Part model, mm, in its own coordinate system. Give positions to 0.01 mm unless a question says otherwise; leave off trailing zeros. Write each loop counter-clockwise with the first axis right and the second up, starting at its lowest first coordinate (ties: lowest second). Pieces come first, ordered by that corner, then holes. Notation, with made-up numbers: M 71.5,-19.75 L 78.5,-19.75 A29 cw 78.5,0.25 Z; hole C -18.5,81 d10. An arc over 180 degrees is marked long. Use CSV: the item, a comma, the result in double quotes. Start each with the question number.
1. Drop a flat-ended pin along its axis: pin 1 Ø3.5 at (x, z) = (-87.1, -54.87) entering from +Y. Give the stop position or say it passes through.
2. Band-saw the part on B-B, the plane x = -20. List the corners of the cut face in (y, z), then the cut area to 3 significant figures.
3. Drill centre lines: line 1 along Z through (x, y) = (71, 1.7); line 2 along X through (y, z) = (5, 5). Where is each one in solid material? Low to high. Write a range as from..to.
4. Band-saw the part on A-A, the plane z = -29.5. List the corners of the cut face in (x, y), then the cut area to 3 significant figures.
5. Band-saw the part on C-C, the plane y = 1.9. List the corners of the cut face in (x, z).
from build123d import *

# Parameters (mm, degrees)
SKETCH_1_W          = 187
SKETCH_1_H          = 114
EXTRUDE_1_DEPTH     = 6
FILLET_1_R          = 3
SKETCH_3_W          = 164.9
SKETCH_3_H          = 101.6
CUT_EXTRUDE_1_DEPTH = 6
SKETCH_6_R          = 1.5
CUT_EXTRUDE_3_DEPTH = 6
SKETCH_7_R          = 2.75
CUT_EXTRUDE_4_DEPTH = 2


with BuildPart() as part:
    # 草图1 → 凸台-拉伸1 (new body)
    with BuildSketch(Plane(origin=(0, 0, 0), x_dir=(1, 0, 0), z_dir=(0, 1, 0))):
        with Locations((0.200214133, 4.065310493)):
            Rectangle(SKETCH_1_W, SKETCH_1_H)
    extrude(amount=EXTRUDE_1_DEPTH)

    # 圆角1
    fillet_1_edges = [part.edges().sort_by_distance(p)[0] for p in [
        (-93.299785867, 3, -61.065310493),
        (93.700214133, 3, -61.065310493),
        (93.700214133, 3, 52.934689507),
        (-93.299785867, 3, 52.934689507),
    ]]
    fillet(fillet_1_edges, radius=FILLET_1_R)

    # 草图3 → 切除-拉伸1 (cut)
    with BuildSketch(Plane(origin=(0, 6, 0), x_dir=(1, 0, 0), z_dir=(0, 1, 0))):
        with Locations((0.200562113, 4.065310493)):
            Rectangle(SKETCH_3_W, SKETCH_3_H)
    extrude(amount=-CUT_EXTRUDE_1_DEPTH, mode=Mode.SUBTRACT)

    # 草图6 → 切除-拉伸3 (cut)
    with BuildSketch(Plane(origin=(0, 6, 0), x_dir=(1, 0, 0), z_dir=(0, 1, 0))):
        with Locations(Location((87.500562113, -46.734892708, 0), (0, 0, 270))):
            Circle(SKETCH_6_R)
        with Locations(Location((87.500562113, 54.865513693, 0), (0, 0, 90))):
            Circle(SKETCH_6_R)
        with Locations(Location((-87.100133848, -46.734892708, 0), (0, 0, 90))):
            Circle(SKETCH_6_R)
        with Locations(Location((-87.100133848, 54.865513693, 0), (0, 0, 270))):
            Circle(SKETCH_6_R)
    extrude(amount=-CUT_EXTRUDE_3_DEPTH, mode=Mode.SUBTRACT)

    # 草图7 → 切除-拉伸4 (cut)
    with BuildSketch(Plane(origin=(0, 6, 0), x_dir=(1, 0, 0), z_dir=(0, 1, 0))):
        with Locations(Location((-87.099785867, 54.865310493, 0), (0, 0, 270))):
            Circle(SKETCH_7_R)
        with Locations(Location((87.500214133, 54.865310493, 0), (0, 0, 90))):
            Circle(SKETCH_7_R)
        with Locations(Location((-87.099785867, -46.734689507, 0), (0, 0, 90))):
            Circle(SKETCH_7_R)
        with Locations(Location((87.500214133, -46.734689507, 0), (0, 0, 270))):
            Circle(SKETCH_7_R)
    extrude(amount=-CUT_EXTRUDE_4_DEPTH, mode=Mode.SUBTRACT)


solid = part.part
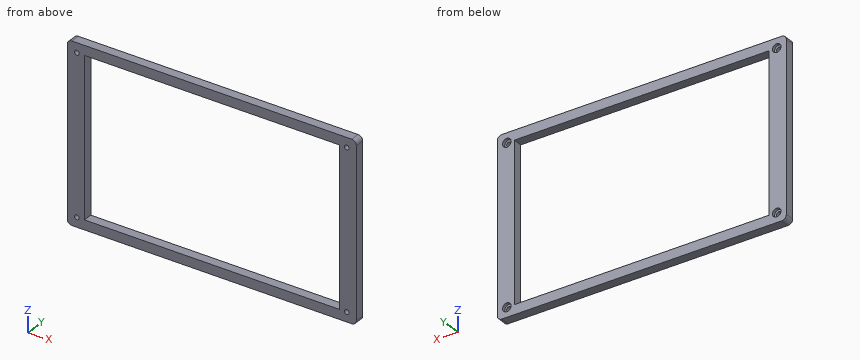
Output:
1,pin 1,"stops at y = 4"
2,outline,"M 0,-61.07 L 6,-61.07 L 6,-54.87 L 0,-54.87 Z; M 0,46.73 L 6,46.73 L 6,52.93 L 0,52.93 Z"
2,area,"74.4 mm²"
3,line 1,"z = -61.07..-54.87, 46.73..52.93"
3,line 2,"x = -93.3..-82.25, 82.65..93.7"
4,outline,"M -93.3,0 L -82.25,0 L -82.25,6 L -93.3,6 Z; M 82.65,0 L 93.7,0 L 93.7,6 L 82.65,6 Z"
4,area,"133 mm²"
5,outline,"M -93.3,-58.07 A3 ccw -90.3,-61.07 L 90.7,-61.07 A3 ccw 93.7,-58.07 L 93.7,49.93 A3 ccw 90.7,52.93 L -90.3,52.93 A3 ccw -93.3,49.93 Z; hole C -87.1,-54.87 d3; hole C -87.1,46.73 d3; hole M -82.25,-54.87 L 82.65,-54.87 L 82.65,46.73 L -82.25,46.73 Z; hole C 87.5,-54.87 d3; hole C 87.5,46.73 d3"
